from build123d import *

# Parameters (mm, degrees)
SKETCH1_W           = 36.1
SKETCH1_H           = 26
SKETCH1_R           = 1.6
BOSS_EXTRUDE1_DEPTH = 1.2
BOSS_EXTRUDE2_DEPTH = 3.5
SKETCH3_W           = 24.5
SKETCH3_H           = 24.5
BOSS_EXTRUDE3_DEPTH = 0.7
BOSS_EXTRUDE5_DEPTH = 4
BOSS_EXTRUDE6_DEPTH = 0.1
SKETCH6_R           = 0.907363589
BOSS_EXTRUDE7_DEPTH = 0.5
SKETCH7_W           = 12
SKETCH7_H           = 15.7
BOSS_EXTRUDE8_DEPTH = 2
SKETCH8_R           = 2.4
BOSS_EXTRUDE9_DEPTH = 7
SKETCH9_R           = 1.6
CUT_EXTRUDE3_DEPTH  = 28.996472992


with BuildPart() as part:
    # Sketch1 → Boss-Extrude1 (new body)
    with BuildSketch(Plane.XY):
        Rectangle(SKETCH1_W, SKETCH1_H)
        with Locations((-15.4, 10.4)):
            Circle(SKETCH1_R, mode=Mode.SUBTRACT)
        with Locations(Location((15.4, 10.4, 0), (0, 0, 180))):
            Circle(SKETCH1_R, mode=Mode.SUBTRACT)
        with Locations((15.4, -10.4)):
            Circle(SKETCH1_R, mode=Mode.SUBTRACT)
        with Locations(Location((-15.4, -10.4, 0), (0, 0, 180))):
            Circle(SKETCH1_R, mode=Mode.SUBTRACT)
    extrude(amount=BOSS_EXTRUDE1_DEPTH)

    # Sketch2 → Boss-Extrude2 (add)
    with BuildSketch(Plane(origin=(0, 0, 0), x_dir=(-1, 0, 0), z_dir=(0, 0, -1))):
        Polygon((-10.35, 12.25), (-12.35, 10.25), (-12.35, -10.25), (-10.35, -12.25), (10.15, -12.25), (12.15, -10.25), (12.15, 10.25), (10.15, 12.25), align=None)
    extrude(amount=BOSS_EXTRUDE2_DEPTH)

    # Sketch3 → Boss-Extrude3 (add)
    with BuildSketch(Plane(origin=(0, 0, -3.5), x_dir=(-1, 0, 0), z_dir=(0, 0, -1))):
        with Locations((-0.1, 0)):
            Rectangle(SKETCH3_W, SKETCH3_H)
    extrude(amount=BOSS_EXTRUDE3_DEPTH)

    # Sketch4 → Boss-Extrude5 (add)
    with BuildSketch(Plane(origin=(0, 0, -4.2), x_dir=(-1, 0, 0), z_dir=(0, 0, -1))):
        with BuildLine():
            Line((10.1, -12.2), (-10.3, -12.2))
            ThreePointArc((-10.3, -12.2), (-11.714213562, -11.614213562), (-12.3, -10.2))
            Line((-12.3, -10.2), (-12.3, 10.2))
            ThreePointArc((-12.3, 10.2), (-11.714213562, 11.614213562), (-10.3, 12.2))
            Line((-10.3, 12.2), (10.1, 12.2))
            ThreePointArc((10.1, 12.2), (11.514213562, 11.614213562), (12.1, 10.2))
            Line((12.1, 10.2), (12.1, -10.2))
            ThreePointArc((12.1, -10.2), (11.514213562, -11.614213562), (10.1, -12.2))
        make_face()
    extrude(amount=BOSS_EXTRUDE5_DEPTH)

    # Sketch5 → Boss-Extrude6 (add)
    with BuildSketch(Plane(origin=(0, 0, -8.2), x_dir=(-1, 0, 0), z_dir=(0, 0, -1))):
        with BuildLine():
            Line((9.5, -11.5), (-9.5, -11.5))
            ThreePointArc((-9.5, -11.5), (-10.914213562, -10.914213562), (-11.5, -9.5))
            Line((-11.5, -9.5), (-11.5, 9.5))
            ThreePointArc((-11.5, 9.5), (-10.914213562, 10.914213562), (-9.5, 11.5))
            Line((-9.5, 11.5), (9.5, 11.5))
            ThreePointArc((9.5, 11.5), (10.914213562, 10.914213562), (11.5, 9.5))
            Line((11.5, 9.5), (11.5, -9.5))
            ThreePointArc((11.5, -9.5), (10.914213562, -10.914213562), (9.5, -11.5))
        make_face()
    extrude(amount=BOSS_EXTRUDE6_DEPTH)

    # Sketch6 → Boss-Extrude7 (add)
    with BuildSketch(Plane(origin=(0, 0, -8.3), x_dir=(-1, 0, 0), z_dir=(0, 0, -1))):
        with Locations((1, 0)):
            Circle(SKETCH6_R)
    extrude(amount=BOSS_EXTRUDE7_DEPTH)

    # Sketch7 → Boss-Extrude8 (add)
    with BuildSketch(Plane.XY.offset(1.2)):
        Rectangle(SKETCH7_W, SKETCH7_H)
    extrude(amount=BOSS_EXTRUDE8_DEPTH)

    # Sketch8 → Boss-Extrude9 (add)
    with BuildSketch(Plane.XY.offset(1.2)):
        with Locations((-15.4, 10.4)):
            Circle(SKETCH8_R)
        with Locations(Location((15.4, 10.4, 0), (0, 0, 180))):
            Circle(SKETCH8_R)
        with Locations((15.4, -10.4)):
            Circle(SKETCH8_R)
        with Locations(Location((-15.4, -10.4, 0), (0, 0, 180))):
            Circle(SKETCH8_R)
    extrude(amount=BOSS_EXTRUDE9_DEPTH)

    # Sketch9 → Cut-Extrude3 (cut, through all)
    with BuildSketch(Plane.XY.offset(8.2)):
        with Locations((-15.4, 10.4)):
            Circle(SKETCH9_R)
        with Locations(Location((-15.4, -10.4, 0), (0, 0, 180))):
            Circle(SKETCH9_R)
        with Locations((15.4, -10.4)):
            Circle(SKETCH9_R)
        with Locations(Location((15.4, 10.4, 0), (0, 0, 180))):
            Circle(SKETCH9_R)
    extrude(amount=-CUT_EXTRUDE3_DEPTH, mode=Mode.SUBTRACT)


solid = part.part
Design review of the part built by this model. Coordinates are the model's own, in mm. A direction names the side the tool comes from. Give positions to 0.01 mm unless a question says otherwise; leave off trailing zeros. Loops run counter-clockwise (first coordinate to the right, second up) from the corner with the lowest first, then second, coordinate; pieces in that order, holes last. Notation, with made-up numbers: (66.5, 82.25) - (106.5, 82.25) arc R11 cw to (106.5, 89.25) - close; hole circle Ø5 at (40.25, -39.75). An arc over 180 degrees is marked (long way). Use CSV: the item, a comma, the result in double quotes. Start each with the question number.
1. Add section D-D (z = -5.75). State the section outline as (x, y) points, plus the area to 3 significant figures.
2. Add section A-A (x = -15.4). State the section outline as (y, z) points.
3. Add section B-B (z = 4.25). State the section outline as (x, y) points, plus the area to 3 significant figures.
4. Machinability: for faces 4 (the cylindrical face through (-0.9, 0.9, -8.5)), 5 (the flat face through (-12, -12, -3.5)), 6 (the flat face through (11.3, 11.3, -1.7)), which of the approach directions +Z, -Z, +X, -X, +Y, -Y give a long, thin tool a straight path to every point of the face, cutting with its end or side? Answer none if there is none.
5. Insertion check: P1, Ø2, axis at x = -10, z = 3, coming from the -Y side; P2, Ø7.5, axis at x = 5.5, y = 0.5, coming from the -Z side; P3, Ø0.6, axis at x = -1, z = 2, coming from the -Y side; P4, Ø0.6, axis at y = -3.5, z = 2, coming from the -X side. Each pin has a flat end and moves straight along its axis. Give the tip position at first contact, or say it passes through.
6. Add section C-C (y = -5.25). State the section outline as (x, z) points, plus the area to 3 significant figures.
7. Draft analysis for pull direction Z (two halves, no side actions). For faces 1 (the flat face through (11.4, -11.2, -1.7)), 2 (the flat face through (-1, 0, -8.8)), 3 (the flat face through (0, 7.85, 2)), state which applies: released by +Z, released by -Z, zero draft, split by the parting line, or undercut.
8. Wall thickness on L1, parallel to Y at x = -15.4, z = 4.5; L2, parallel to Z at x = 16, y = -8; L3, parallel to X at y = -2.5, z = -3.75: over which ranges is each line inside the solid? List them lowest first.
Results found:
1,outline,"(-12.1, -10.2) arc R2 ccw to (-10.1, -12.2) - (10.3, -12.2) arc R2 ccw to (12.3, -10.2) - (12.3, 10.2) arc R2 ccw to (10.3, 12.2) - (-10.1, 12.2) arc R2 ccw to (-12.1, 10.2) - close"
1,area,"592 mm²"
2,outline,"(-13, 0) - (-12, 0) - (-12, 8.2) - (-12.8, 8.2) - (-12.8, 1.2) - (-13, 1.2) - close; (-8.8, 0) - (8.8, 0) - (8.8, 8.2) - (8, 8.2) - (8, 1.2) - (-8, 1.2) - (-8, 8.2) - (-8.8, 8.2) - close; (12, 0) - (13, 0) - (13, 1.2) - (12.8, 1.2) - (12.8, 8.2) - (12, 8.2) - close"
3,outline,"circle Ø4.8 at (-15.4, -10.4); circle Ø4.8 at (-15.4, 10.4); circle Ø4.8 at (15.4, -10.4); circle Ø4.8 at (15.4, 10.4); hole circle Ø3.2 at (-15.4, -10.4); hole circle Ø3.2 at (-15.4, 10.4); hole circle Ø3.2 at (15.4, -10.4); hole circle Ø3.2 at (15.4, 10.4)"
3,area,"40.2 mm²"
4,face 4,"-Z"
4,face 5,"-X, -Y"
4,face 6,"+X, +Y"
5,P1,"passes through"
5,P2,"stops at z = -8.3"
5,P3,"stops at y = -7.85"
5,P4,"stops at x = -6"
6,outline,"(-18.05, 0) - (-12.15, 0) - (-12.15, -4.2) - (-12.1, -4.2) - (-12.1, -8.2) - (-11.5, -8.2) - (-11.5, -8.3) - (11.5, -8.3) - (11.5, -8.2) - (12.3, -8.2) - (12.3, -4.2) - (12.35, -4.2) - (12.35, 0) - (18.05, 0) - (18.05, 1.2) - (6, 1.2) - (6, 3.2) - (-6, 3.2) - (-6, 1.2) - (-18.05, 1.2) - close"
6,area,"270 mm²"
7,face 1,"undercut"
7,face 2,"released by -Z"
7,face 3,"zero draft"
8,L1,"y = -12.8 to -12, -8.8 to -8, 8 to 8.8, 12 to 12.8"
8,L2,"z = 0 to 1.2"
8,L3,"x = -12.15 to 12.35"
